Here's how the part is built. I have some questions about the finished solid (model axes, mm). A direction names the side the tool comes from. Give positions to 0.01 mm unless a question says otherwise; leave off trailing zeros. Loops run counter-clockwise (first coordinate to the right, second up) from the corner with the lowest first, then second, coordinate; pieces in that order, holes last. Notation, with made-up numbers: (10, 40.25) - (25, 40.25) arc R23 cw to (25, 50.25) - close; hole circle Ø5 at (-11, -25.5). An arc over 180 degrees is marked (long way). Use a Markdown table: item, result.
from build123d import *

# Parameters (mm, degrees)
F0_R     = 10.15
F1_DEPTH = 19.8
F2_R     = 15
F3_R     = 5
F4_R     = 5
F5_R     = 2
F6_R     = 2
F7_W     = 7.765233
F7_H     = 2.4
F8_DEPTH = 28


with BuildPart() as f1:
    # F0 (on Top) → F1 (new body)
    with BuildSketch(Plane.XY):
        Polygon((-56.2, 17.5), (-56.2, -17.5), (-49.2, -17.5), (-49.2, 10.5), (-35, 10.5), (-35, -17.5), (49.886581, -17.5), (49.886581, 17.5), align=None)
        with Locations((29.886581, 0)):
            Circle(F0_R, mode=Mode.SUBTRACT)
    extrude(amount=F1_DEPTH)

    # F2
    f2_edges = [f1.edges().sort_by_distance(p)[0] for p in [
        (49.886581, 17.5, 9.9),
        (49.886581, -17.5, 9.9),
    ]]
    fillet(f2_edges, radius=F2_R)

    # F3
    f3_edges = [f1.edges().sort_by_distance(p)[0] for p in [
        (-35, -17.5, 9.9),
    ]]
    fillet(f3_edges, radius=F3_R)

    # F4
    f4_edges = [f1.edges().sort_by_distance(p)[0] for p in [
        (-56.2, 17.5, 9.9),
    ]]
    fillet(f4_edges, radius=F4_R)

    # F5
    f5_edges = [f1.edges().sort_by_distance(p)[0] for p in [
        (-49.2, -17.5, 9.9),
        (-56.2, -17.5, 9.9),
    ]]
    fillet(f5_edges, radius=F5_R)

    # F6
    f6_edges = [f1.edges().sort_by_distance(p)[0] for p in [
        (-49.2, 10.5, 9.9),
        (-35, 10.5, 9.9),
    ]]
    fillet(f6_edges, radius=F6_R)

    # F7 (on face) → F8 (cut, through all)
    with BuildSketch(Plane.XZ.offset(17.5)):
        with Locations((-52.807339, 11.1)):
            Rectangle(F7_W, F7_H)
        with Locations((-52.807339, 8.7)):
            Rectangle(F7_W, F7_H)
    extrude(amount=-F8_DEPTH, mode=Mode.SUBTRACT)


solid = f1.part
(1) Suppose I cut it at C-C on x = 36.5. Write out the boundary of the cut face in (y, z).
A:
| item | result |
|---|---|
| outline | (-17.41, 0) - (-7.7, 0) - (-7.7, 19.8) - (-17.41, 19.8) - close; (7.7, 0) - (17.41, 0) - (17.41, 19.8) - (7.7, 19.8) - close |
(2) Suppose I cut it at D-D on z = 1.75. Write out the boundary of the cut face in (x, y), plus the area to 3 significant figures.
A:
| item | result |
|---|---|
| outline | (-56.2, -15.5) arc R2 ccw to (-54.2, -17.5) - (-51.2, -17.5) arc R2 ccw to (-49.2, -15.5) - (-49.2, 8.5) arc R2 cw to (-47.2, 10.5) - (-37, 10.5) arc R2 cw to (-35, 8.5) - (-35, -12.5) arc R5 ccw to (-30, -17.5) - (34.89, -17.5) arc R15 ccw to (49.89, -2.5) - (49.89, 2.5) arc R15 ccw to (34.89, 17.5) - (-51.2, 17.5) arc R5 ccw to (-56.2, 12.5) - close; hole circle Ø20.3 at (29.89, 0) |
| area | 2,880 mm2 |
(3) Suppose I cut it at B-B on y = 0. Write out the boundary of the cut face in (x, z), plus the area to 3 significant figures.
A:
| item | result |
|---|---|
| outline | (-56.2, 0) - (-49.2, 0) - (-49.2, 7.5) - (-56.2, 7.5) - close; (-56.2, 12.3) - (-49.2, 12.3) - (-49.2, 19.8) - (-56.2, 19.8) - close; (-35, 0) - (19.74, 0) - (19.74, 19.8) - (-35, 19.8) - close; (40.04, 0) - (49.89, 0) - (49.89, 19.8) - (40.04, 19.8) - close |
| area | 1,380 mm2 |
(4) Suppose I cut it at A-A on z = 10. Write out the boundary of the cut face in (x, y).
A:
| item | result |
|---|---|
| outline | (-56.2, 10.5) - (-48.92, 10.5) - (-48.92, 9.51) arc R2 cw to (-47.2, 10.5) - (-37, 10.5) arc R2 cw to (-35, 8.5) - (-35, -12.5) arc R5 ccw to (-30, -17.5) - (34.89, -17.5) arc R15 ccw to (49.89, -2.5) - (49.89, 2.5) arc R15 ccw to (34.89, 17.5) - (-51.2, 17.5) arc R5 ccw to (-56.2, 12.5) - close; hole circle Ø20.3 at (29.89, 0) |
(5) Will these pins go through, and if not, where does the flat tip stop? pin 1 (6 mm diameter, centred on y = -6.5, z = 2, fed in from +X); pin 2 (2.5 mm diameter, centred on y = -7, z = 15.5, fed in from +X); pin 3 (16 mm diameter, centred on x = 29.89, y = 0, fed in from -Z); pin 4 (8 mm diameter, centred on x = -40, z = 12.5, fed in from -Y).
A:
| item | result |
|---|---|
| pin 1 | x = 49.85 |
| pin 2 | x = 49.53 |
| pin 3 | through |
| pin 4 | y = 10.23 |
(6) If I drill on line 1 (X direction, y = -9, z = 1); line 2 (X direction, y = 1, z = 5); line 3 (Y direction, x = -34.5, z = 11.5), over which ranges is the centre line in solid material (lowest first)?
A:
| item | result |
|---|---|
| line 1 | -56.2 to -49.2, -35 to 25.19, 34.58 to 48.41 |
| line 2 | -56.2 to -49.2, -35 to 19.79, 39.99 to 49.89 |
| line 3 | -14.68 to 17.5 |
(7) On a 3-axis mill with a long thin cutter (end or side, diameter ignored), from which of +Z, -Z, +X, -X, +Y, -Y can I reach the whole of each face in a straight line? I mean faces 1 (the face through (-35.6, 9.93, 10.04)), 2 (the face through (49.887, 0, 10)), 3 (the face through (-53, -4, 12.3)). Say none if no direction works.
A:
| item | result |
|---|---|
| face 1 | +Z, -Z, -Y |
| face 2 | +Z, -Z, +X, +Y, -Y |
| face 3 | -X, -Y |
(8) We'd pull the mould along Z, two halves only. Please class faces 4 (the face through (45.4, 13.2, 10)), 5 (the face through (-53, 10.5, 10)): pulls with the +Z half, pulls with the -Z half, needs draft (parallel to the pull), parting line crosses it, or undercut.
A:
| item | result |
|---|---|
| face 4 | needs draft |
| face 5 | undercut |
